```python
from build123d import *

# Parameters (mm, degrees)
SKETCH1_R           = 22.225
SKETCH1_R_2         = 2.159
BOSS_EXTRUDE1_DEPTH = 2.54
BOSS_EXTRUDE2_START = -2.54
SKETCH1_4_R         = 9.525
BOSS_EXTRUDE2_DEPTH = 2.54


with BuildPart() as part:
    # Sketch1 → Boss-Extrude1 (new body)
    with BuildSketch(Plane(origin=(0, 0, 0), x_dir=(1, 0, 0), z_dir=(0, 1, 0))):
        with Locations(Location((0, 0, 0), (0, 0, 270))):
            Circle(SKETCH1_R)
        with BuildLine():
            Line((-2.5, -1.658312395), (-2.5, 1.658312395))
            ThreePointArc((-2.5, 1.658312395), (3, 0), (-2.5, -1.658312395))
        make_face(mode=Mode.SUBTRACT)
        with Locations(Location((0, -14.21564213, 0), (0, 0, 270))):
            Circle(SKETCH1_R_2, mode=Mode.SUBTRACT)
        with Locations(Location((14.21564213, 0, 0), (0, 0, 270))):
            Circle(SKETCH1_R_2, mode=Mode.SUBTRACT)
        with Locations(Location((-14.21564213, 0, 0), (0, 0, 270))):
            Circle(SKETCH1_R_2, mode=Mode.SUBTRACT)
        with Locations(Location((0, 14.21564213, 0), (0, 0, 270))):
            Circle(SKETCH1_R_2, mode=Mode.SUBTRACT)
    extrude(amount=BOSS_EXTRUDE1_DEPTH)

    # Sketch1_4 → Boss-Extrude2 (add)
    with BuildSketch(Plane(origin=(0, 0, 0), x_dir=(1, 0, 0), z_dir=(0, 1, 0)).offset(BOSS_EXTRUDE2_START)):
        with Locations(Location((0, 0, 0), (0, 0, 270))):
            Circle(SKETCH1_4_R)
        with BuildLine():
            Line((-2.5, -1.658312395), (-2.5, 1.658312395))
            ThreePointArc((-2.5, 1.658312395), (3, 0), (-2.5, -1.658312395))
        make_face(mode=Mode.SUBTRACT)
    extrude(amount=BOSS_EXTRUDE2_DEPTH)


solid = part.part
```
Work out the finished part from the listing and answer in its coordinate system (mm). A direction names the side the tool comes from. Give positions to 0.01 mm unless a question says otherwise; leave off trailing zeros. Order: outer loops, then holes, each group sorted by start corner. A loop starts at its lowest first (then second) coordinate and runs counter-clockwise, first axis right, second up.
1. Section D-D, the plane y = -1.4 is taken. Determine the outline of the cut face in (x, z) (3 decimals), and give its area (3 significant figures).
Result sheet:
outline: circle Ø19.05 at (0, 0); hole (-2.5, -1.658) arc R3 ccw (long way) to (-2.5, 1.658) - close
area: 258 mm2
2. The mould has two halves that part along X. Classify faces 3 (the flat face through (-2.5, 0, 0)), 4 (the cylindrical face through (18.74, 1.25, 11.95)), 5 (the flat face through (2.3, -2.54, -2.3)): released by +X, released by -X, zero draft, split by the parting line, or undercut.
Result sheet:
face 3: undercut
face 4: split by the parting line
face 5: zero draft
3. Section B-B, the plane x = 0 is taken. Determine the outline of the cut face in (y, z) (3 decimals), and give its area (3 significant figures).
Result sheet:
outline: (-2.54, -9.525) - (0, -9.525) - (0, -12.057) - (2.54, -12.057) - (2.54, -3) - (-2.54, -3) - close; (-2.54, 3) - (2.54, 3) - (2.54, 12.057) - (0, 12.057) - (0, 9.525) - (-2.54, 9.525) - close; (0, -22.225) - (2.54, -22.225) - (2.54, -16.375) - (0, -16.375) - close; (0, 16.375) - (2.54, 16.375) - (2.54, 22.225) - (0, 22.225) - close
area: 109 mm2
4. Section C-C, the plane z = 14 is taken. Determine the outline of the cut face in (x, y), and give its area (3 significant figures).
Result sheet:
outline: (-17.26, 0) - (-2.15, 0) - (-2.15, 2.54) - (-17.26, 2.54) - close; (2.15, 0) - (17.26, 0) - (17.26, 2.54) - (2.15, 2.54) - close
area: 76.8 mm2
5. For faces 1 (the cylindrical face through (-5.796, -1.288, -7.559)), 2 (the flat face through (-5, 2.54, 0)), determine the directions among +Z, -Z, +X, -X, +Y, -Y from which every point of the face is accessible in a straight line to the end or side of a thin tool.
Result sheet:
face 1: -Y
face 2: +Z, -Z, +X, -X, +Y
6. Section A-A, the plane z = 0 is taken. Determine the outline of the cut face in (x, y) (3 decimals).
Result sheet:
outline: (-22.225, 0) - (-16.375, 0) - (-16.375, 2.54) - (-22.225, 2.54) - close; (-12.057, 0) - (-9.525, 0) - (-9.525, -2.54) - (-2.5, -2.54) - (-2.5, 2.54) - (-12.057, 2.54) - close; (3, -2.54) - (9.525, -2.54) - (9.525, 0) - (12.057, 0) - (12.057, 2.54) - (3, 2.54) - close; (16.375, 0) - (22.225, 0) - (22.225, 2.54) - (16.375, 2.54) - close
7. Each of these flat-tipped pins is pushed along its axis until it touches: P1, Ø1.5, axis at x = 11, z = -11.5, coming from the -Y side; P2, Ø5.5, axis at x = 0, z = 0, coming from the -Y side; P3, Ø1.5, axis at y = 0, z = 7, coming from the +X side; P4, Ø2.5, axis at y = 0.5, z = -1, coming from the +X side (3 decimals). Where does it stop, or does it pass through?
Result sheet:
P1: stops at y = 0
P2: stops at y = -2.54
P3: stops at x = 21.33
P4: stops at x = 22.225
8. Straight lines are drawn through the part: L1, parallel to X at y = 1.3, z = 0 (3 decimals); L2, parallel to Y at x = -20, z = -3; L3, parallel to Z at x = 1.5, y = -0.7. For each, find the intervals that lie inside material, in ascending order.
Result sheet:
L1: x = -22.225 to -16.375, -12.057 to -2.5, 3 to 12.057, 16.375 to 22.225
L2: y = 0 to 2.54
L3: z = -9.41 to -2.6, 2.6 to 9.41
